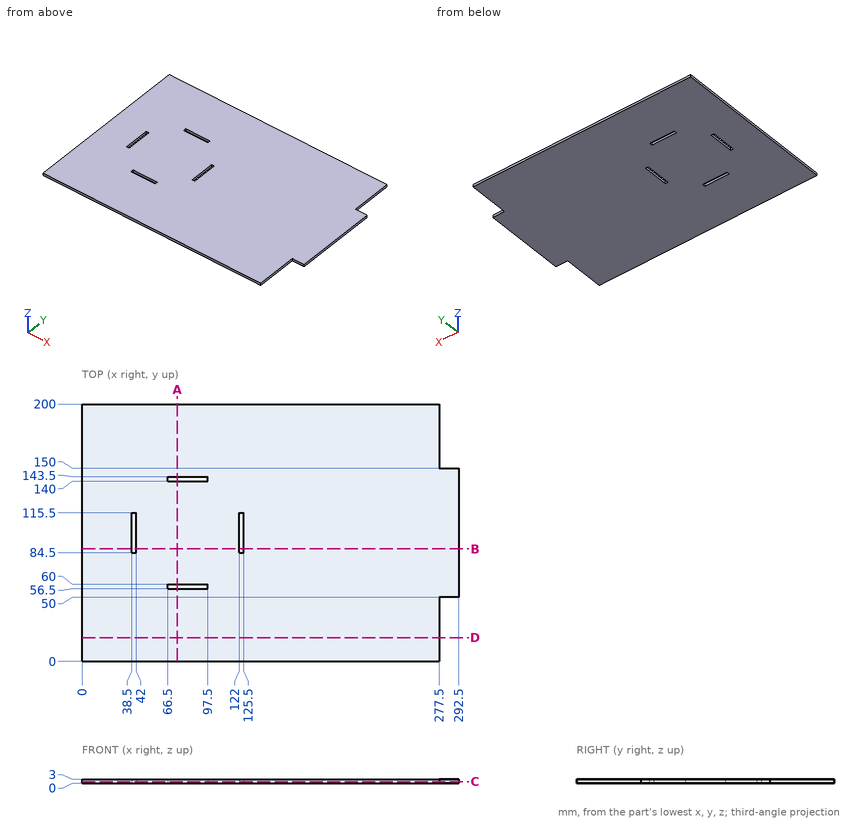
Can you work these out from the drawing? Everything is in mm from the part's minimum corner. Coordinates: 2 decimals unless noted, no trailing zeros. Write each loop counter-clockwise with the first axis right and the second up, starting at its lowest first coordinate (ties: lowest second). Pieces come first, ordered by that corner, then holes. Notation, with made-up numbers: (-20, 54.25) -> (-5, 54.25) arc R28 ccw to (-5, 84.25) -> close; hole circle Ø11 at (63, 21.5). An arc over 180 degrees is marked (long way). Write each question's results on one line, items separated by ' | '. Start each with the question number.
Q1. Imagine slicing it at A-A (x = 74). Write out the boundary of the cut face in (y, z), then the cut area to 3 significant figures.
Q2. If I drill on probe 1 along X at (y, z) = (107, 1.75); probe 2 along Y at (x, z) = (72, 0.6); probe 3 along Y at (x, z) = (280, 2.7), over which ranges is the centre line in solid material (lowest first)?
Q3. I'm going to push flat-ended pins straight in: pin 1 (0.9 mm diameter, centred on x = 284, z = 1, fed in from +Y); pin 2 (1.5 mm diameter, centred on x = 288.5, z = 2, fed in from -Y); pin 3 (1.5 mm diameter, centred on y = 28.5, z = 2, fed in from +X). Where does each tip first touch, or does it pass through?
Q4. Imagine slicing it at D-D (y = 18.5). Write out the boundary of the cut face in (x, z).
Q5. Imagine slicing it at C-C (z = 1.3). Write out the boundary of the cut face in (x, y).
Q6. Imagine slicing it at B-B (y = 87.5). Write out the boundary of the cut face in (x, z).
Taken from the geometry:
1) outline: (0, 0) -> (56.5, 0) -> (56.5, 3) -> (0, 3) -> close; (60, 0) -> (140, 0) -> (140, 3) -> (60, 3) -> close; (143.5, 0) -> (200, 0) -> (200, 3) -> (143.5, 3) -> close | area: 579 mm^2
2) probe 1: x = 0 to 38.5, 42 to 122, 125.5 to 292.5 | probe 2: y = 0 to 56.5, 60 to 140, 143.5 to 200 | probe 3: y = 50 to 150
3) pin 1: stops at y = 150 | pin 2: stops at y = 50 | pin 3: stops at x = 277.5
4) outline: (0, 0) -> (277.5, 0) -> (277.5, 3) -> (0, 3) -> close
5) outline: (0, 0) -> (277.5, 0) -> (277.5, 50) -> (292.5, 50) -> (292.5, 150) -> (277.5, 150) -> (277.5, 200) -> (0, 200) -> close; hole (38.5, 84.5) -> (42, 84.5) -> (42, 115.5) -> (38.5, 115.5) -> close; hole (66.5, 56.5) -> (97.5, 56.5) -> (97.5, 60) -> (66.5, 60) -> close; hole (66.5, 140) -> (97.5, 140) -> (97.5, 143.5) -> (66.5, 143.5) -> close; hole (122, 84.5) -> (125.5, 84.5) -> (125.5, 115.5) -> (122, 115.5) -> close
6) outline: (0, 0) -> (38.5, 0) -> (38.5, 3) -> (0, 3) -> close; (42, 0) -> (122, 0) -> (122, 3) -> (42, 3) -> close; (125.5, 0) -> (292.5, 0) -> (292.5, 3) -> (125.5, 3) -> close
